Work out the finished part from the listing and answer in its coordinate system (mm). Coordinates: 2 decimals unless noted, no trailing zeros. Loops run counter-clockwise (first coordinate to the right, second up) from the corner with the lowest first, then second, coordinate; pieces in that order, holes last.
```python
from build123d import *

# Parameters (mm, degrees)
BOSS_EXTRUDE1_DEPTH = 6.35
SKETCH2_W           = 10.16
SKETCH2_H           = 6.326695662
BOSS_EXTRUDE2_DEPTH = 54.61
SKETCH3_R           = 1.651
CUT_EXTRUDE1_DEPTH  = 6.35
SKETCH4_R           = 1.651
CUT_EXTRUDE2_DEPTH  = 22.606
FILLET1_R           = 3.81


with BuildPart() as part:
    # Sketch1 → Boss-Extrude1 (new body)
    with BuildSketch(Plane(origin=(0, 0, 0), x_dir=(1, 0, 0), z_dir=(0, 1, 0))):
        with BuildLine():
            Line((-66.04, 0), (-76.2, 0))
            ThreePointArc((-76.2, 0), (-68.233584612, -33.920759587), (-46.000054305, -60.748950641))
            Line((-46.000054305, -60.748950641), (-39.866713731, -52.649090555))
            ThreePointArc((-39.866713731, -52.649090555), (-59.135773331, -29.397991642), (-66.04, 0))
        make_face()
    extrude(amount=BOSS_EXTRUDE1_DEPTH)

    # Sketch2 → Boss-Extrude2 (add)
    with BuildSketch(Plane(origin=(0, 0, 0), x_dir=(-1, 0, 0), z_dir=(0, 0, -1))):
        with Locations((71.12, 3.186652169)):
            Rectangle(SKETCH2_W, SKETCH2_H)
    extrude(amount=BOSS_EXTRUDE2_DEPTH)

    # Sketch3 → Cut-Extrude1 (cut)
    with BuildSketch(Plane(origin=(0, 6.35, 0), x_dir=(1, 0, 0), z_dir=(0, 1, 0))):
        with Locations(Location((-71.12, 51.435, 0), (0, 0, 270))):
            Circle(SKETCH3_R)
    extrude(amount=-CUT_EXTRUDE1_DEPTH, mode=Mode.SUBTRACT)

    # Sketch4 → Cut-Extrude2 (cut)
    with BuildSketch(Plane(origin=(0, 6.35, 0), x_dir=(1, 0, 0), z_dir=(0, 1, 0))):
        with Locations(Location((-45.464590295, -54.782351668, 0), (0, 0, 270))):
            Circle(SKETCH4_R)
    extrude(amount=-CUT_EXTRUDE2_DEPTH, mode=Mode.SUBTRACT)

    # Fillet1
    fillet1_edges = [part.edges().sort_by_distance(p)[0] for p in [
        (-66.04, 3.186652169, -54.61),
        (-76.2, 3.186652169, -54.61),
    ]]
    fillet(fillet1_edges, radius=FILLET1_R)


solid = part.part
```
1. A cutting plane is placed at C-C, the plane z = -30. Give the vertices of the cut face in (x, y), then the cut area to 3 significant figures.
2. A cutting plane is placed at D-D, the plane x = -51. Give the vertices of the cut face in (y, z).
3. A cutting plane is placed at A-A, the plane y = 5. Give the vertices of the cut face in (x, z) (3 decimals), then the cut area to 3 significant figures.
4. Each of these flat-tipped pins is pushed along its axis until it touches: P1, Ø1.9, axis at y = 4.5, z = -36, coming from the +X side; P2, Ø3, axis at x = -72.5, z = -15, coming from the -Y side; P3, Ø3, axis at x = -71.12, z = -51.435, coming from the -Y side; P4, Ø1, axis at y = 2, z = 17.5, coming from the +X side. Where does it stop, or does it pass through?
5. Determine the mould class of faces 1 (the cylindrical face through (-68.45, 3.13, 33.48)), 2 (the flat face through (-61, 0, 28)), 3 (the cylindrical face through (-75.054, 3.231, -53.524)), 4 (the cylindrical face through (-69.483, 3.231, -51.65)) for opening direction Z: released by +Z, released by -Z, zero draft, split by the parting line, or undercut.
6. Straight lines are drawn through the part: probe 1 along X at (y, z) = (4.25, -3); probe 2 along Y at (x, z) = (-70, -1); probe 3 along X at (y, z) = (1.75, 54). For each, find the intervals that lie inside material, in ascending order.
Answers below:
1. outline: (-76.2, 0.02) - (-66.04, 0.02) - (-66.04, 6.35) - (-76.2, 6.35) - close
1. area: 64.3 mm2
2. outline: (0, 41.96) - (6.35, 41.96) - (6.35, 56.62) - (0, 56.62) - close
3. outline: (-76.2, -50.8) arc R3.81 ccw to (-72.39, -54.61) - (-69.85, -54.61) arc R3.81 ccw to (-66.04, -50.8) - (-66.04, 0) arc R66.04 cw to (-39.867, 52.649) - (-46, 60.749) arc R76.2 ccw to (-76.2, 0) - close; hole circle Ø3.302 at (-71.12, -51.435); hole circle Ø3.302 at (-45.465, 54.782)
3. area: 1,200 mm2
4. P1: stops at x = -66.04
4. P2: stops at y = 0.02
4. P3: passes through
4. P4: stops at x = -63.54
5. face 1: released by +Z
5. face 2: zero draft
5. face 3: released by -Z
5. face 4: undercut
6. probe 1: x = -76.2 to -66.04
6. probe 2: y = 0.02 to 6.35
6. probe 3: x = -53.76 to -46.92, -44.01 to -40.89
